Here's the drawing with two shaded views (mm, measured from the low corner). I have some questions. A direction names the side the tool comes from. Give positions to 0.01 mm unless a question says otherwise; leave off trailing zeros. Order: outer loops, then holes, each group sorted by start corner. A loop starts at its lowest first (then second) coordinate and runs counter-clockwise, first axis right, second up. Notation, with made-up numbers: M 59.5,59.25 L 65.5,59.25 A11 cw 65.5,65.25 Z; hole C 53.25,68 d3. An arc over 180 degrees is marked long. One line per question, with ' | ' between items. Start each with the question number.
1) If we section it at A-A, the plane x = 21: Please give me the cut outline in (y, z), plus the area to 3 significant figures.
2) If we section it at C-C, the plane y = 14: Please give me the cut outline in (x, z).
3) For the marked faces 5, 6, 7 and 8, which set-ups out of +Z, -Z, +X, -X, +Y, -Y let a thin tool reach every point of the face, with its end or its side?
4) If we section it at D-D, the plane z = 7: Please give me the cut outline in (x, y).
5) Thinking about a two-plate mould opening in Y: for the marked faces 1, 2, 3 and 4, which applies, +Y half, -Y half, draft (parallel to the pull), parting line (faces both ways), or undercut?
6) If we section it at B-B, the plane z = 9.25: Please give me the cut outline in (x, y).
7) Please list where these lines run through material, in increasing order: line 1 along Y through (x, z) = (26, 3.25); line 2 along Y through (x, z) = (26.5, 3.5); line 3 along X through (y, z) = (6.5, 6). Write a range as [from, to].
8) I'm going to push flat-ended pins straight in: pin 1 Ø4 at (x, z) = (31, 2) entering from -Y; pin 2 Ø5 at (y, z) = (17, 1.5) entering from -X. Where does each tip first touch, or does it pass through?
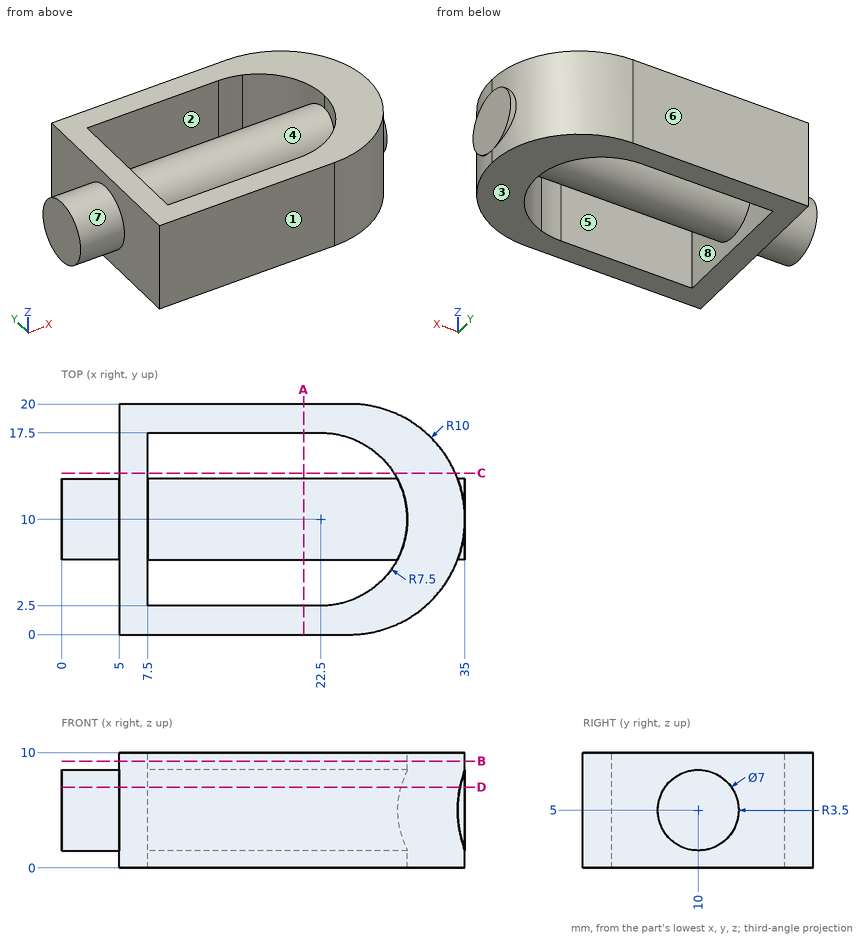
Results found:
1) outline: M 0,0 L 2.5,0 L 2.5,10 L 0,10 Z; C 10,5 d7; M 17.5,0 L 20,0 L 20,10 L 17.5,10 Z | area: 88.5 mm²
2) outline: M 5,0 L 7.5,0 L 7.5,10 L 5,10 Z; M 28.84,0 L 34.17,0 L 34.17,10 L 28.84,10 Z
3) face 5: +Z, -Z | face 6: +Z, -Z, +X, -X, +Y | face 7: -X | face 8: none
4) outline: M 0,7.13 L 5,7.13 L 5,0 L 25,0 A10 ccw 34.58,7.13 L 35,7.13 L 35,12.87 L 34.58,12.87 A10 ccw 25,20 L 5,20 L 5,12.87 L 0,12.87 Z; hole M 7.5,2.5 L 22.5,2.5 A7.5 ccw 29.43,7.13 L 7.5,7.13 Z; hole M 7.5,12.87 L 29.43,12.87 A7.5 ccw 22.5,17.5 L 7.5,17.5 Z
5) face 1: -Y half | face 2: undercut | face 3: draft | face 4: undercut
6) outline: M 5,0 L 25,0 A10 ccw 25,20 L 5,20 Z; hole M 7.5,2.5 L 22.5,2.5 A7.5 ccw 22.5,17.5 L 7.5,17.5 Z
7) line 1: y = [0.05, 3.37], [6.97, 13.03], [16.63, 19.95] | line 2: y = [0.11, 3.66], [6.84, 13.16], [16.34, 19.89] | line 3: x = [5, 7.5], [29.13, 34.37]
8) pin 1: stops at y = 0.83 | pin 2: stops at x = 5
